Autodesk Inventor part; units mm, degrees
ref_plane "YZ Plane" through (0, 0, 0) normal (1, 0, 0) x (0, 1, 0)
ref_plane "XZ Plane" through (0, 0, 0) normal (0, 1, 0) x (-1, 0, 0)
ref_plane "XY Plane" through (0, 0, 0) normal (0, 0, 1) x (1, 0, 0)
sketch "Sketch1" plane through (0, 0, 0) normal (0, 1, 0) x (-1, 0, 0)
  line L0 (47.9425, 45.085) -> (-47.9425, 45.085)
  line L1 (-47.9425, 45.085) -> (-47.9425, -45.085)
  line L2 (-47.9425, -45.085) -> (47.9425, -45.085)
  line L3 (47.9425, -45.085) -> (47.9425, 45.085)
  line L4 (47.9425, 45.085) -> (-47.9425, -45.085) construction
  line L5 (-47.9425, 45.085) -> (47.9425, -45.085) construction
  circle A0 centre (42.8625, 36.195) radius 1.5875
  circle A1 centre (42.8625, -36.195) radius 1.5875
  circle A2 centre (-42.8625, -40.005) radius 1.5875
  circle A3 centre (-42.8625, 40.005) radius 1.5875
  point P0 (0, 0)
  dimension "d0" = 90.17
  dimension "d1" = 95.885
  dimension "d2" = 5.08
  dimension "d3" = 5.08
  dimension "d4" = 5.08
  dimension "d5" = 8.89
  dimension "d6" = 8.89
  dimension "d7" = 5.08
  dimension "d8" = 3.175
  dimension "d9" = 3.175
  dimension "d10" = 3.175
  dimension "d11" = 3.175
extrude "Extrusion1" add sketch "Sketch1" along normal mid plane 1.6
sketch "Sketch2" plane through (0, -0.8, 0) normal (0, -1, 0) x (1, 0, 0)
  circle A0 centre (36.4425, 20.415) radius 1.6
  circle A1 centre (13.4425, 20.415) radius 1.6
  circle A2 centre (36.4425, -37.585) radius 1.6
  circle A3 centre (13.4425, -37.585) radius 1.6
  circle A4 centre (-34.4425, -37.085) radius 1.6
  circle A5 centre (-9.6925, -37.085) radius 1.6
  circle A6 centre (-34.5675, -1.385) radius 1.1
  circle A7 centre (-9.5675, -1.385) radius 1.1
  point P0 (0, 0)
  dimension "d14" = 9.5675
  dimension "d15" = 34.5675
  dimension "d16" = 9.6925
  dimension "d17" = 34.4425
  dimension "d18" = 1.385
  dimension "d19" = 2.2
  dimension "d20" = 1.385
  dimension "d21" = 37.085
  dimension "d22" = 37.085
  dimension "d23" = 33.0002
  dimension "d24" = 3.2
  dimension "d25" = 3.2
  dimension "d26" = 20.415
  dimension "d28" = 13.4425
  dimension "d29" = 36.4425
  dimension "d30" = 37.585
  dimension "d31" = 20.415
  dimension "d32" = 19.8
  dimension "d34" = 58
extrude "Extrusion2" cut sketch "Sketch2" against normal up to surface (1.6 mm away)
equation "\"d9\" = d8"
equation "\"d10\" = d8"
equation "\"d11\" = d8"
properties part number "PC 104 size and hole model_Hermes_Top_Mount_V1" material "FR-4"
Check sheet for the modelled part. Datum: model origin and axes. Units: mm. Coordinates: 2 decimals unless noted, no trailing zeros.
1) Gauge pin test, flat end, axial feed: pin 1 (2.5 mm diameter, centred on x = 42.86, z = 40.01, fed in from -Y). Record the tip position at first contact, or that the pin passes through.
2) Release check for a two-part mould opening along X. For faces 1 (the face through (1, 0.8, 1)), 2 (the face through (11.844, -0.011, -37.515)) record: released by +X, released by -X, zero draft, split by the parting line, or undercut.
3) Material ranges on probe 1 along Z at (x, y) = (43, -0.25) (3 decimals); probe 2 along Z at (x, y) = (42, 0.55) (3 decimals); probe 3 along X at (y, z) = (-0.05, -39), recorded low to high.
Check sheet entries:
1. pin 1: passes through
2. face 1: zero draft
2. face 2: undercut
3. probe 1: z = -45.085 to -41.587, -38.423 to 38.423, 41.587 to 45.085
3. probe 2: z = -45.085 to -41.338, -38.672 to 38.672, 41.338 to 45.085
3. probe 3: x = -47.94 to 12.7, 14.19 to 35.7, 37.19 to 41.63, 44.09 to 47.94
